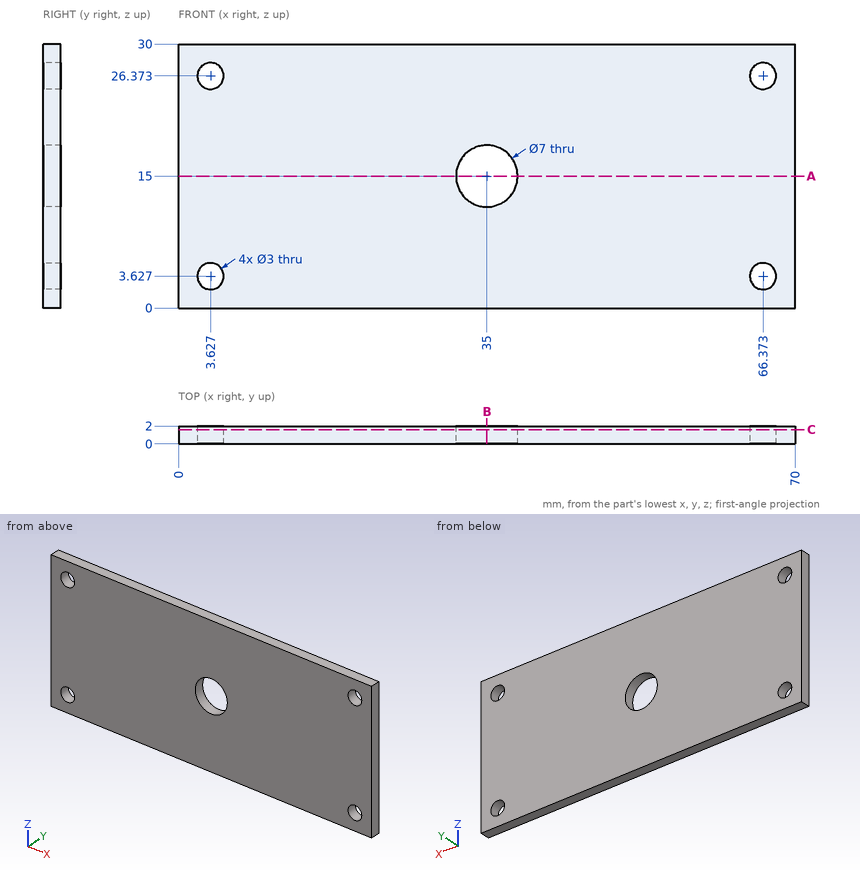
Check sheet for the drawn part. Datum: minimum x, y, z corner. Units: mm. Give positions to 0.01 mm unless a question says otherwise; leave off trailing zeros. Loops run counter-clockwise (first coordinate to the right, second up) from the corner with the lowest first, then second, coordinate; pieces in that order, holes last.
1) Thickness scan on line 1 along X through (y, z) = (1.25, 26.5); line 2 along Z through (x, y) = (67, 0.5) (1 decimal); line 3 along Z through (x, y) = (65, 1.5) (1 decimal). Record the ranges inside material, lowest first.
2) Sectioned sample at C-C, the plane y = 1.6. Enter the section's corners in (x, z), then the cut area to 3 significant figures.
3) Depth check by flat-ended pin: pin 1 Ø4 at (x, z) = (35, 15) entering from +Y; pin 2 Ø4 at (x, z) = (66.37, 3.63) entering from +Y. Enter the tip coordinate at first touch or a pass-through.
4) Sectioned sample at A-A, the plane z = 15. Enter the section's corners in (x, y).
5) Sectioned sample at B-B, the plane x = 35. Enter the section's corners in (y, z).
Answers:
1. line 1: x = 0 to 2.13, 5.12 to 64.88, 67.87 to 70
1. line 2: z = 0 to 2.3, 5 to 25, 27.7 to 30
1. line 3: z = 0 to 3, 4.2 to 25.8, 27 to 30
2. outline: (0, 0) - (70, 0) - (70, 30) - (0, 30) - close; hole circle Ø3 at (3.63, 3.63); hole circle Ø3 at (3.63, 26.37); hole circle Ø7 at (35, 15); hole circle Ø3 at (66.37, 3.63); hole circle Ø3 at (66.37, 26.37)
2. area: 2,030 mm2
3. pin 1: passes through
3. pin 2: stops at y = 2
4. outline: (0, 0) - (31.5, 0) - (31.5, 2) - (0, 2) - close; (38.5, 0) - (70, 0) - (70, 2) - (38.5, 2) - close
5. outline: (0, 0) - (2, 0) - (2, 11.5) - (0, 11.5) - close; (0, 18.5) - (2, 18.5) - (2, 30) - (0, 30) - close
